Source: three-view drawing plus pictorial views. Frame: mm from the lowest corner of the part. Coordinates: 2 decimals unless noted, no trailing zeros. Loops run counter-clockwise (first coordinate to the right, second up) from the corner with the lowest first, then second, coordinate; pieces in that order, holes last.
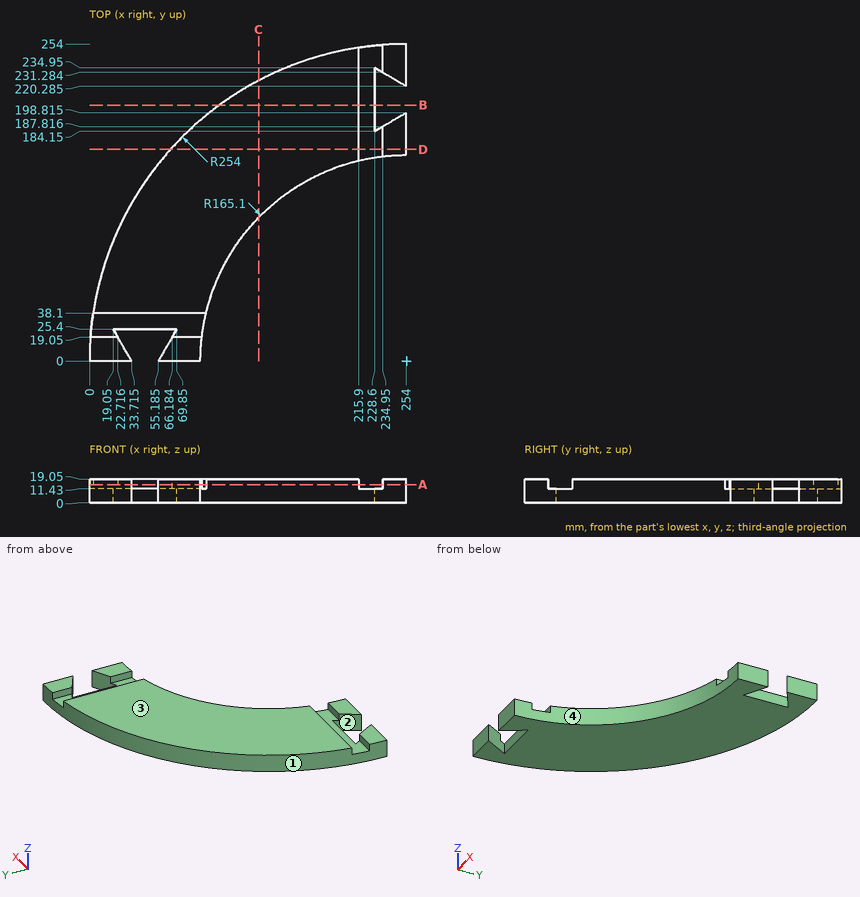
Q1. Draft query along X for the marked faces 1, 2, 3 and 4. Return one class per face: +X half, -X half, draft (parallel to the pull), parting line (faces both ways), or undercut.
Q2. Section D-D, the plane y = 169.5. Return the cut outline in (x, z).
Q3. Section A-A, the plane z = 14.5. Count the separate pieces of the cut face and the enclosed holes in it, plus the area to 3 significant figures.
Q4. Contact query for flat-ended pins moving along their axis: pin 1 Ø3.5 at (y, z) = (216, 5.5) entering from +X; pin 2 Ø3.5 at (x, z) = (34.5, 7) entering from -Y; pin 3 Ø8.5 at (y, z) = (178, 13.5) entering from -X (1 decimal); pin 4 Ø1.5 at (x, z) = (36.5, 15.5) entering from +Y. Output: stop coordinate, or through.
Q5. Section C-C, the plane x = 135.5. Return the cut outline in (y, z).
Q6. Line query: line 1 along Y through (x, z) = (237, 16.5); line 2 along Z through (x, y) = (32.5, 35.5); line 3 along Y through (x, z) = (23.5, 17) (1 decimal). Output: solid intervals per line, ascending.
Q7. Section B-B, the plane y = 205. Return the cut outline in (x, z), plus the area to 3 significant figures.
Derived:
1. face 1: -X half
1. face 2: undercut
1. face 3: draft
1. face 4: +X half
2. outline: (64.83, 0) - (254, 0) - (254, 19.05) - (234.95, 19.05) - (234.95, 11.43) - (215.9, 11.43) - (215.9, 19.05) - (64.83, 19.05) - close
3. separate pieces: 5
3. enclosed holes: 0
3. area: 24,600 mm2
4. pin 1: stops at x = 228.6
4. pin 2: stops at y = 0
4. pin 3: stops at x = 68.7
4. pin 4: stops at y = 132.42
5. outline: (114.96, 0) - (224.66, 0) - (224.66, 19.05) - (114.96, 19.05) - close
6. line 1: y = 164.22 to 189, 230.1 to 253.43
6. line 2: z = 0 to 11.43
6. line 3: y = 0 to 17.7, 38.1 to 106.7
7. outline: (104.03, 0) - (228.6, 0) - (228.6, 11.43) - (215.9, 11.43) - (215.9, 19.05) - (104.03, 19.05) - close
7. area: 2,280 mm2
